The model under review builds one solid part; all positions refer to its coordinate system, in mm. Coordinates: 2 decimals unless noted, no trailing zeros. Answer as a JSON object with one key per item and string values.
```python
from build123d import *

# Parameters (mm, degrees)
SKETCH6_R           = 2.1
BOSS_EXTRUDE1_DEPTH = 483


with BuildPart() as part:
    # Sketch6 → Boss-Extrude1 (new body)
    with BuildSketch(Plane.XY):
        with BuildLine():
            Line((-3.4, -2.339339828), (-3.4, 2.339339828))
            Line((-3.4, 2.339339828), (-6.560660172, 5.5))
            Line((-6.560660172, 5.5), (-8.2, 5.5))
            Line((-8.2, 5.5), (-8.2, 2.89))
            Line((-8.2, 2.89), (-8.31, 2.89))
            Line((-8.31, 2.89), (-9.768614357, 4.348614357))
            ThreePointArc((-9.768614357, 4.348614357), (-9.939864831, 4.604908803), (-10, 4.907228714))
            Line((-10, 4.907228714), (-10, 8.5))
            ThreePointArc((-10, 8.5), (-9.560660172, 9.560660172), (-8.5, 10))
            Line((-8.5, 10), (-4.907228714, 10))
            ThreePointArc((-4.907228714, 10), (-4.604908803, 9.939864831), (-4.348614357, 9.768614357))
            Line((-4.348614357, 9.768614357), (-2.89, 8.31))
            Line((-2.89, 8.31), (-2.89, 8.2))
            Line((-2.89, 8.2), (-5.5, 8.2))
            Line((-5.5, 8.2), (-5.5, 6.560660172))
            Line((-5.5, 6.560660172), (-2.339339828, 3.4))
            Line((-2.339339828, 3.4), (2.339339828, 3.4))
            Line((2.339339828, 3.4), (5.5, 6.560660172))
            Line((5.5, 6.560660172), (5.5, 8.2))
            Line((5.5, 8.2), (2.89, 8.2))
            Line((2.89, 8.2), (2.89, 8.31))
            Line((2.89, 8.31), (4.348614357, 9.768614357))
            ThreePointArc((4.348614357, 9.768614357), (4.604908803, 9.939864831), (4.907228714, 10))
            Line((4.907228714, 10), (8.5, 10))
            ThreePointArc((8.5, 10), (9.560660172, 9.560660172), (10, 8.5))
            Line((10, 8.5), (10, 4.907228714))
            ThreePointArc((10, 4.907228714), (9.939864831, 4.604908803), (9.768614357, 4.348614357))
            Line((9.768614357, 4.348614357), (8.31, 2.89))
            Line((8.31, 2.89), (8.2, 2.89))
            Line((8.2, 2.89), (8.2, 5.5))
            Line((8.2, 5.5), (6.560660172, 5.5))
            Line((6.560660172, 5.5), (3.4, 2.339339828))
            Line((3.4, 2.339339828), (3.4, -2.339339828))
            Line((3.4, -2.339339828), (6.560660172, -5.5))
            Line((6.560660172, -5.5), (8.2, -5.5))
            Line((8.2, -5.5), (8.2, -2.89))
            Line((8.2, -2.89), (8.31, -2.89))
            Line((8.31, -2.89), (9.768614357, -4.348614357))
            ThreePointArc((9.768614357, -4.348614357), (9.939864831, -4.604908803), (10, -4.907228714))
            Line((10, -4.907228714), (10, -8.5))
            ThreePointArc((10, -8.5), (9.560660172, -9.560660172), (8.5, -10))
            Line((8.5, -10), (4.907228714, -10))
            ThreePointArc((4.907228714, -10), (4.604908803, -9.939864831), (4.348614357, -9.768614357))
            Line((4.348614357, -9.768614357), (2.89, -8.31))
            Line((2.89, -8.31), (2.89, -8.2))
            Line((2.89, -8.2), (5.5, -8.2))
            Line((5.5, -8.2), (5.5, -6.560660172))
            Line((5.5, -6.560660172), (2.339339828, -3.4))
            Line((2.339339828, -3.4), (-2.339339828, -3.4))
            Line((-2.339339828, -3.4), (-5.5, -6.560660172))
            Line((-5.5, -6.560660172), (-5.5, -8.2))
            Line((-5.5, -8.2), (-2.89, -8.2))
            Line((-2.89, -8.2), (-2.89, -8.31))
            Line((-2.89, -8.31), (-4.348614357, -9.768614357))
            ThreePointArc((-4.348614357, -9.768614357), (-4.604908803, -9.939864831), (-4.907228714, -10))
            Line((-4.907228714, -10), (-8.5, -10))
            ThreePointArc((-8.5, -10), (-9.560660172, -9.560660172), (-10, -8.5))
            Line((-10, -8.5), (-10, -4.907228714))
            ThreePointArc((-10, -4.907228714), (-9.939864831, -4.604908803), (-9.768614357, -4.348614357))
            Line((-9.768614357, -4.348614357), (-8.31, -2.89))
            Line((-8.31, -2.89), (-8.2, -2.89))
            Line((-8.2, -2.89), (-8.2, -5.5))
            Line((-8.2, -5.5), (-6.560660172, -5.5))
            Line((-6.560660172, -5.5), (-3.4, -2.339339828))
        make_face()
        Circle(SKETCH6_R, mode=Mode.SUBTRACT)
        Polygon((-7.66, 6.57), (-6.57, 7.66), (-6.57, 8.2), (-8.2, 8.2), (-8.2, 6.57), align=None, mode=Mode.SUBTRACT)
        Polygon((8.2, 6.57), (7.66, 6.57), (6.57, 7.66), (6.57, 8.2), (8.2, 8.2), align=None, mode=Mode.SUBTRACT)
        Polygon((7.66, -6.57), (6.57, -7.66), (6.57, -8.2), (8.2, -8.2), (8.2, -6.57), align=None, mode=Mode.SUBTRACT)
        Polygon((-8.2, -6.57), (-7.66, -6.57), (-6.57, -7.66), (-6.57, -8.2), (-8.2, -8.2), align=None, mode=Mode.SUBTRACT)
    extrude(amount=-BOSS_EXTRUDE1_DEPTH)


solid = part.part
```
(1) For pin 1 Ø6 at (y, z) = (1, -83) entering from -X; pin 2 Ø3 at (x, z) = (-2, -326.5) entering from +Y; pin 3 Ø3.5 at (y, z) = (1, -254.5) entering from +X; pin 4 Ø5 at (x, y) = (0.5, 6) entering from -Z, all flat-tipped, find the tip position at first contact; note any pin that passes through.
Results list:
{"pin 1": "x = -9.42", "pin 2": "y = 8.92", "pin 3": "x = 3.81", "pin 4": "through"}
(2) Add section A-A on z = -426.5. Count the separate pieces of the cut face and the enclosed holes in it, and give its area (3 significant figures).
Results list:
{"separate pieces": "1", "enclosed holes": "5", "area": "152 mm²"}
(3) Wall thickness on line 1 along X through (y, z) = (0.5, -155); line 2 along Y through (x, z) = (0, -351.5); line 3 along Y through (x, z) = (5.25, -299.5): over which ranges is each line inside the solid? List them lowest first. Write a range as from..to.
Results list:
{"line 1": "-3.4..-2.04, 2.04..3.4", "line 2": "-3.4..-2.1, 2.1..3.4", "line 3": "-10..-8.2, -6.31..-4.19, 4.19..6.31, 8.2..10"}
